from build123d import *

# Parameters (mm, degrees)
BOSS_EXTRUDE1_DEPTH = 7
SKETCH2_R           = 22.5
BOSS_EXTRUDE2_DEPTH = 3
CUT_EXTRUDE1_DEPTH  = 101.307028667
SKETCH4_R           = 17.5
CUT_EXTRUDE2_DEPTH  = 101.560926806
SKETCH5_R           = 18.5
CUT_EXTRUDE3_DEPTH  = 7


with BuildPart() as part:
    # Sketch1 → Boss-Extrude1 (new body)
    with BuildSketch(Plane.XY):
        with BuildLine():
            Line((-56.635632328, 13), (67.516685226, 13))
            ThreePointArc((67.516685226, 13), (90, 0), (67.516685226, -13))
            Line((67.516685226, -13), (-56.635632328, -13))
            ThreePointArc((-56.635632328, -13), (-97.5, 0), (-56.635632328, 13))
        make_face()
    extrude(amount=BOSS_EXTRUDE1_DEPTH)

    # Sketch2 → Boss-Extrude2 (add)
    with BuildSketch(Plane.XY.offset(7)):
        with Locations(Location((-75, 0, 0), (0, 0, 324.705605323))):
            Circle(SKETCH2_R)
    extrude(amount=BOSS_EXTRUDE2_DEPTH)

    # Sketch3 → Cut-Extrude1 (cut, through all)
    with BuildSketch(Plane.XY.offset(7)):
        Polygon((82.5, 0), (78.75, 6.495190528), (71.25, 6.495190528), (67.5, 0), (71.25, -6.495190528), (78.75, -6.495190528), align=None)
    extrude(amount=-CUT_EXTRUDE1_DEPTH, mode=Mode.SUBTRACT)

    # Sketch4 → Cut-Extrude2 (cut, through all)
    with BuildSketch(Plane.XY.offset(10)):
        with Locations((-75, 0)):
            Circle(SKETCH4_R)
    extrude(amount=-CUT_EXTRUDE2_DEPTH, mode=Mode.SUBTRACT)

    # Sketch5 → Cut-Extrude3 (cut)
    with BuildSketch(Plane.XY):
        with Locations((-75, 0)):
            Circle(SKETCH5_R)
    extrude(amount=CUT_EXTRUDE3_DEPTH, mode=Mode.SUBTRACT)


solid = part.part
Can you work these out from the model? Positions are in its coordinate system, mm. A direction names the side the tool comes from. Give positions to 0.01 mm unless a question says otherwise; leave off trailing zeros. Write each loop counter-clockwise with the first axis right and the second up, starting at its lowest first coordinate (ties: lowest second). Pieces come first, ordered by that corner, then holes. Notation, with made-up numbers: (59.5, 57) -> (100.5, 57) arc R6 ccw to (100.5, 61) -> close; hole circle Ø9 at (60.5, 18.5). An arc over 180 degrees is marked (long way). Answer as a JSON object with one key per item and string values. Group by question number.
Item 1: Please list where these lines run through material, in increasing order: line 1 (Y direction, x = -75, z = 4.25); line 2 (Y direction, x = -75, z = 8.3); line 3 (X direction, y = -4.5, z = 4.25). Write a range as [from, to].
Item 2: I'm going to push flat-ended pins straight in: P1, Ø5.5, axis at x = 76, z = 2, coming from the -Y side; P2, Ø1.5, axis at x = 0, y = 3.5, coming from the +Z side; P3, Ø4, axis at x = -65.5, z = 5, coming from the -Y side; P4, Ø1, axis at x = 49, y = -14, coming from the -Z side. Where does each tip first touch, or does it pass through?
Item 3: Suppose I cut it at D-D (y = 9). Please give me the cut outline in (x, z), plus the area to 3 significant figures.
Item 4: For faces 4 (the face through (5, 13, 3)), 5 (the face through (6, -13, 3)), 6 (the face through (-93.482, 0.813, 3.451)), 7 (the face through (75, 6.495, 4)), which set-ups out of +Z, -Z, +X, -X, +Y, -Y let a thin tool reach every point of the face, with its end or its side?
Item 5: Suppose I cut it at A-A (x = 75). Please give me the cut outline in (y, z).
Item 6: Suppose I cut it at C-C (z = 1.75). Please give me the cut outline in (x, y), plus the area to 3 significant figures.
Item 7: We'd pull the mould along X, two halves only. Please class faces 1 (the face through (18, 0, 0)), 2 (the face through (75, -6.495, 4)), 3 (the face through (-58.834, -6.703, 8.521)): +X half, -X half, draft (parallel to the pull), parting line (faces both ways), or undercut.
Item 8: Suppose I cut it at B-B (y = 2). Please give me the cut outline in (x, z).
Findings:
{
 "1": {"line 1": "y = [-22.5, -18.5], [18.5, 22.5]", "line 2": "y = [-22.5, -17.5], [17.5, 22.5]", "line 3": "x = [-97.05, -92.94], [-57.06, 70.1], [79.9, 89.31]"},
 "2": {"P1": "stops at y = -15", "P2": "stops at z = 7", "P3": "stops at y = -21.21", "P4": "passes through"},
 "3": {"outline": "(-95.62, 0) -> (-91.16, 0) -> (-91.16, 7) -> (-90.01, 7) -> (-90.01, 10) -> (-95.62, 10) -> close; (-59.99, 7) -> (-58.84, 7) -> (-58.84, 0) -> (87, 0) -> (87, 7) -> (-54.38, 7) -> (-54.38, 10) -> (-59.99, 10) -> close", "area": "1,090 mm²"},
 "4": {"face 4": "+Z, -Z, +Y", "face 5": "+Z, -Z, -Y", "face 6": "-Z", "face 7": "+Z, -Z"},
 "5": {"outline": "(-15, 0) -> (-6.5, 0) -> (-6.5, 7) -> (-15, 7) -> close; (6.5, 0) -> (15, 0) -> (15, 7) -> (6.5, 7) -> close"},
 "6": {"outline": "(-56.64, -13) -> (67.52, -13) arc R15 ccw (long way) to (67.52, 13) -> (-56.64, 13) arc R22.5 ccw (long way) to start; hole circle Ø37 at (-75, 0); hole (67.5, 0) -> (71.25, -6.5) -> (78.75, -6.5) -> (82.5, 0) -> (78.75, 6.5) -> (71.25, 6.5) -> close", "area": "4,090 mm²"},
 "7": {"face 1": "draft", "face 2": "undercut", "face 3": "undercut"},
 "8": {"outline": "(-97.41, 0) -> (-93.39, 0) -> (-93.39, 7) -> (-92.39, 7) -> (-92.39, 10) -> (-97.41, 10) -> close; (-57.61, 7) -> (-56.61, 7) -> (-56.61, 0) -> (68.65, 0) -> (68.65, 7) -> (-52.59, 7) -> (-52.59, 10) -> (-57.61, 10) -> close; (81.35, 0) -> (89.87, 0) -> (89.87, 7) -> (81.35, 7) -> close"}
}
